Solid Edge part; units mm, degrees
sketch "Sketch1" plane through (0, 0, 0) normal (0, -1, 0) x (1, 0, 0)
  line L0 (0, 0) -> (9, 0)
  line L1 (9, 0) -> (7.5, 3)
  line L2 (7.5, 3) -> (0, 3)
  dimension "D1" = 9
  dimension "D2" = 7.5
revolve "RevolvedProtrusion1" add sketch "Sketch1" angle 360 about axis through (0, 0, 3) along (0, 0, -1)
sketch "Sketch2" plane through (0, 0, 3) normal (0, 0, 1) x (1, 0, 0)
  line L0 (-0.5, -4) -> (0.5, -4)
  line L1 (0.5, -4) -> (0.5, 4)
  line L2 (0.5, 4) -> (-0.5, 4)
  line L3 (-0.5, 4) -> (-0.5, -4)
  dimension "D1" = 0.5
  dimension "D2" = 0.5
extrude "Cutout1" cut sketch "Sketch2" against normal blind 0.5
fillet "main_rounds" radius 0.25 6 edges at (-9, 0, 0) (-7.5, 0, 3) (0.5, 0, 3) (0, -4, 3) (-0.5, 0, 3) (0, 4, 3)
properties material "Polyethylene, low density"
Geometry: final body of the model. Coordinates: model frame, mm. Give positions to 0.01 mm unless a question says otherwise; leave off trailing zeros. Loops run counter-clockwise (first coordinate to the right, second up) from the corner with the lowest first, then second, coordinate; pieces in that order, holes last. Notation, with made-up numbers: (26.25, 32.5) - (76.25, 32.5) arc R19 cw to (76.25, 48.5) - close; hole circle Ø3 at (47, -36.75). An arc over 180 degrees is marked (long way). Answer as CSV lines item,"result". Start each with the question number.
1. Draft query along X for faces 1 (the face through (7.29, -2.3, 2.71)), 2 (the face through (0, 0, 0)), 3 (the face through (0, 0, 2.5)). Return one class per face: released by +X, released by -X, zero draft, split by the parting line, or undercut.
2. Section D-D, the plane z = 0.6. Return loops of the section in (x, y).
3. Section C-C, the plane z = 1.6. Return loops of the section in (x, y).
4. Ray query, L1, parallel to Z at x = 0, y = -2.5; L2, parallel to X at y = 6.25, z = 1.05; L3, parallel to Y at x = -4.75, z = 0.7. Return the intervals inside material, ascending.
5. Pin query (flat end, axial travel): P1, Ø2, axis at x = -3, y = 3, coming from the -Z side; P2, Ø0.5, axis at x = 0, y = 1, coming from the +Z side; P3, Ø1, axis at x = -3, z = 0.5, coming from the +Y side. Return the tip coordinate at first contact, or that it passes through.
6. Section B-B, the plane x = 0. Return loops of the section in (y, z), plus the area to 3 significant figures.
7. Section A-A, the plane y = 0. Return loops of the section in (x, z).
Answers:
1,face 1,"split by the parting line"
1,face 2,"zero draft"
1,face 3,"undercut"
2,outline,"circle Ø17.4 at (0, 0)"
3,outline,"circle Ø16.4 at (0, 0)"
4,L1,"z = 0 to 2.5"
4,L2,"x = -5.72 to 5.72"
4,L3,"y = -7.23 to 7.23"
5,P1,"stops at z = 0"
5,P2,"stops at z = 2.5"
5,P3,"stops at y = 8.47"
6,outline,"(-8.82, 0.36) arc R0.25 ccw to (-8.6, 0) - (8.6, 0) arc R0.25 ccw to (8.82, 0.36) - (7.57, 2.86) arc R0.25 ccw to (7.35, 3) - (4.25, 3) arc R0.25 ccw to (4, 2.75) - (4, 2.5) - (-4, 2.5) - (-4, 2.75) arc R0.25 ccw to (-4.25, 3) - (-7.35, 3) arc R0.25 ccw to (-7.57, 2.86) - close"
6,area,"45.4 mm2"
7,outline,"(-8.82, 0.36) arc R0.25 ccw to (-8.6, 0) - (8.6, 0) arc R0.25 ccw to (8.82, 0.36) - (7.57, 2.86) arc R0.25 ccw to (7.35, 3) - (0.75, 3) arc R0.25 ccw to (0.5, 2.75) - (0.5, 2.5) - (-0.5, 2.5) - (-0.5, 2.75) arc R0.25 ccw to (-0.75, 3) - (-7.35, 3) arc R0.25 ccw to (-7.57, 2.86) - close"
